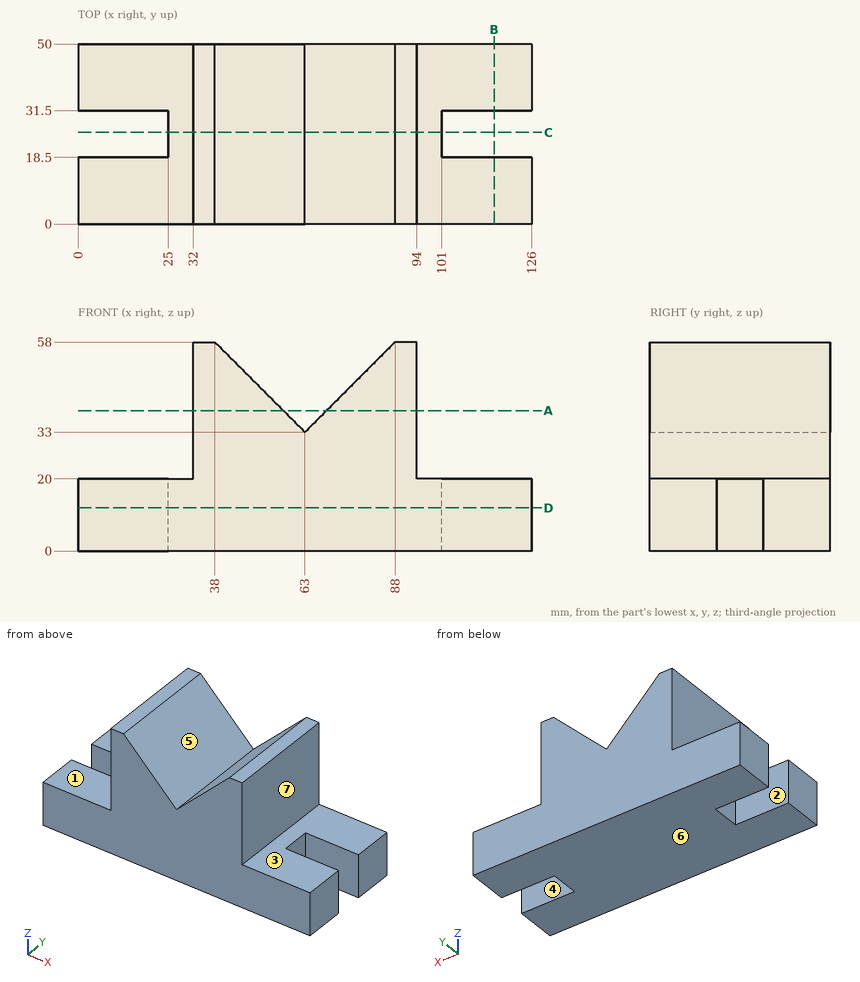
Geometry: see drawing. Coordinates: mm, zero at the bounding-box minimum. A direction names the side the tool comes from. Round coordinates to 2 decimals unless told otherwise and drop trailing zeros. Loops run counter-clockwise (first coordinate to the right, second up) from the corner with the lowest first, then second, coordinate; pieces in that order, holes last. Notation, with made-up numbers: (43.5, 56) - (54.5, 56) arc R22 cw to (54.5, 85) - close; hole circle Ø6 at (-30, 37.25). An arc over 180 degrees is marked (long way). Use CSV: the item, a comma, the result in double quotes.
Q1. Ray query, line 1 along X through (y, z) = (28.5, 8); line 2 along Z through (x, y) = (96, 37); line 3 along X through (y, z) = (46, 23.5). Return the intervals inside material, ascending.
Reported:
line 1,"25 to 101"
line 2,"0 to 20"
line 3,"32 to 94"
Q2. Pin query (flat end, axial travel): pin 1 Ø6.5 at (y, z) = (25, 9.5) entering from +X; pin 2 Ø4 at (y, z) = (37, 42.5) entering from +X; pin 3 Ø11.5 at (y, z) = (17.5, 38.5) entering from -X. Return the tip coordinate at first contact, or that it passes through.
Reported:
pin 1,"x = 101"
pin 2,"x = 94"
pin 3,"x = 32"
Q3. Section query A-A, the plane z = 39. Output: boundary loops of the cut face in (x, y), then the cut area to 3 significant figures.
Reported:
outline,"(32, 0) - (57, 0) - (57, 50) - (32, 50) - close; (69, 0) - (94, 0) - (94, 50) - (69, 50) - close"
area,"2,500 mm^2"
Q4. Reachability of the marked faces 1, 2, 3 and 4 from +Z, -Z, +X, -X, +Y, -Y: full face, straight path, thin tool, end or side. Return the list, or none.
Reported:
face 1,"+Z, -X, +Y, -Y"
face 2,"+Z, -Z, -X"
face 3,"+Z, +X, +Y, -Y"
face 4,"+Z, -Z, +X"
Q5. Section query B-B, the plane x = 115.5. Output: boundary loops of the cut face in (y, z).
Reported:
outline,"(0, 0) - (18.5, 0) - (18.5, 20) - (0, 20) - close; (31.5, 0) - (50, 0) - (50, 20) - (31.5, 20) - close"
Q6. Section query C-C, the plane y = 25.5. Output: boundary loops of the cut face in (x, z).
Reported:
outline,"(25, 0) - (101, 0) - (101, 20) - (94, 20) - (94, 58) - (88, 58) - (63, 33) - (38, 58) - (32, 58) - (32, 20) - (25, 20) - close"
Q7. Mould query, pull axis X, two halves, no side actions, for the marked faces 5, 6 and 7. Classes: pulls with the +X half, pulls with the -X half, needs draft (parallel to the pull), parting line crosses it, or undercut.
Reported:
face 5,"undercut"
face 6,"needs draft"
face 7,"pulls with the +X half"
Q8. Section query D-D, the plane z = 12. Output: boundary loops of the cut face in (x, y), then the cut area to 3 significant figures.
Reported:
outline,"(0, 0) - (126, 0) - (126, 18.5) - (101, 18.5) - (101, 31.5) - (126, 31.5) - (126, 50) - (0, 50) - (0, 31.5) - (25, 31.5) - (25, 18.5) - (0, 18.5) - close"
area,"5,650 mm^2"
